Model file for the job. Use its own axes, mm. A direction names the side the tool comes from. Give positions to 0.01 mm unless a question says otherwise; leave off trailing zeros. Write each loop counter-clockwise with the first axis right and the second up, starting at its lowest first coordinate (ties: lowest second). Pieces come first, ordered by that corner, then holes. Notation, with made-up numbers: (-17.75, 36) - (-13.75, 36) arc R22 ccw to (-13.75, 42) - close; hole circle Ø3 at (4, -1). An arc over 180 degrees is marked (long way). Use a Markdown table: item, result. Add a question column.
Autodesk Inventor part; units mm, degrees
ref_plane "YZ Plane" through (0, 0, 0) normal (1, 0, 0) x (0, 1, 0)
ref_plane "XZ Plane" through (0, 0, 0) normal (0, 1, 0) x (-1, 0, 0)
ref_plane "XY Plane" through (0, 0, 0) normal (0, 0, 1) x (1, 0, 0)
sketch "Sketch1" plane through (0, 0, 0) normal (0, 0, 1) x (1, 0, 0)
  line L0 (-18.415, 5.9563) -> (18.415, 5.9563)
  line L1 (18.415, 5.9563) -> (18.415, -5.9563)
  line L2 (18.415, -5.9563) -> (-18.415, -5.9563)
  line L3 (-18.415, -5.9563) -> (-18.415, 5.9563)
  line L4 (-18.415, 5.9563) -> (18.415, -5.9563) construction
  line L5 (18.415, 5.9563) -> (-18.415, -5.9563) construction
  point P0 (0, 0)
  dimension "d0" = 36.83
  dimension "d1" = 11.9126
extrude "Extrusion1" add sketch "Sketch1" along normal blind 6.35
sketch "Sketch2" plane through (0, 0, 6.35) normal (0, 0, 1) x (1, 0, 0)
  line L0 (-18.415, 5.9563) -> (-18.415, -5.9563)
  line L1 (-18.415, 0) -> (18.415, 0)
  line L2 (18.415, -5.9563) -> (18.415, 5.9563)
  line L3 (-18.415, 0) -> (-20.6375, 0)
  line L4 (-18.415, 0) -> (-12.065, 0)
  circle A0 centre (-12.065, 0) radius 2.3241
  circle A1 centre (0.635, 0) radius 2.3241
  circle A2 centre (13.335, 0) radius 2.3241
  line L5 (-13.716, 2.286) -> (-10.414, 2.286)
  line L6 (-9.779, 1.651) -> (-9.779, -1.651)
  line L7 (-10.414, -2.286) -> (-13.716, -2.286)
  line L8 (-14.351, -1.651) -> (-14.351, 1.651)
  line L9 (-14.351, 2.286) -> (-9.779, -2.286) construction
  line L10 (-9.779, 2.286) -> (-14.351, -2.286) construction
  line L11 (11.684, 2.286) -> (14.986, 2.286)
  line L12 (15.621, 1.651) -> (15.621, -1.651)
  line L13 (14.986, -2.286) -> (11.684, -2.286)
  line L14 (11.049, -1.651) -> (11.049, 1.651)
  line L15 (11.049, 2.286) -> (15.621, -2.286) construction
  line L16 (15.621, 2.286) -> (11.049, -2.286) construction
  arc A3 (-13.716, 2.286) -> (-14.351, 1.651) centre (-13.716, 1.651) ccw
  arc A4 (-9.779, 1.651) -> (-10.414, 2.286) centre (-10.414, 1.651) ccw
  arc A5 (-10.414, -2.286) -> (-9.779, -1.651) centre (-10.414, -1.651) ccw
  arc A6 (-14.351, -1.651) -> (-13.716, -2.286) centre (-13.716, -1.651) ccw
  arc A7 (11.684, 2.286) -> (11.049, 1.651) centre (11.684, 1.651) ccw
  arc A8 (15.621, 1.651) -> (14.986, 2.286) centre (14.986, 1.651) ccw
  arc A9 (14.986, -2.286) -> (15.621, -1.651) centre (14.986, -1.651) ccw
  arc A10 (11.049, -1.651) -> (11.684, -2.286) centre (11.684, -1.651) ccw
  point P0 (0, 0)
  point P1 (-9.779, -0.4191)
  point P2 (-9.7409, 0)
  point P3 (-9.779, 0)
  dimension "d5" = 6.35
  dimension "d6" = 4.6482
  dimension "d9" = 12.7
  dimension "d16" = 4.572
  dimension "d17" = 4.572
  dimension "d18" = 4.572
  dimension "d19" = 4.572
  dimension "d20" = 0.635
extrude "Extrusion2" add sketch "Sketch2" along normal blind 1.5875 contours L8 A0 L5 L6 L1 | L1 L6 A0 L7 L8 | L8 A3 L5 A0 | A0 L7 A6 L8 | L1 A0 L6 | L5 A4 L6 A0 | A0 L6 A5 L7 | L14 A2 L11 L12 L1 | L1 L12 A2 L13 L14 | L14 A7 L11 A2 | A2 L13 A10 L14 | A2 L11 A8 L12 | L12 A9 L13 A2 picked at (-9.772, -0.2331)
extrude "Extrusion3" cut sketch "Sketch2" against normal through all contours A1 L1 | L1 A1
sketch "Sketch9" plane through (-18.415, 5.9563, 0) normal (0, 1, 0) x (1, 0, 0)
  line L0 (0, 0) -> (36.83, 0)
  line L1 (0, -6.35) -> (36.83, -6.35)
  line L2 (0, 0) -> (22.225, 0)
  line L3 (22.225, 0) -> (22.225, -6.35)
  line L4 (22.225, -6.35) -> (0, -6.35)
  line L5 (0, -6.35) -> (0, 0)
  point P0 (18.415, 0)
  dimension "d45" = 22.225
extrude "Extrusion9" add sketch "Sketch9" along normal blind 24.13
sketch "Sketch10" plane through (0, 0, 0) normal (0, 0, -1) x (-1, 0, 0)
  line L0 (-18.415, 5.9563) -> (-3.81, 5.9563)
  line L1 (18.415, 30.0863) -> (-3.81, 30.0863)
  arc A0 (-3.81, 5.9563) -> (-3.81, 30.0863) centre (-3.81, 18.0213) ccw
  line L2 (-3.81, 30.0863) -> (-3.81, 5.9563)
  point P0 (0, 0)
extrude "Extrusion10" cut sketch "Sketch10" against normal blind 19.05
fillet "Fillet7" radius 0.381 1 edges at (3.81, 30.0863, 3.175)
fillet "Fillet8" radius 3.175 4 edges at (-18.415, 30.0863, 3.175) (18.415, 5.9563, 3.175) (18.415, -5.9563, 3.175) (-18.415, -5.9563, 3.175)
sketch "Sketch11" plane through (0, 0, 0) normal (0, 0, -1) x (-1, 0, 0)
  circle A0 centre (-0.635, 0) radius 2.3241
  circle A1 centre (-0.635, 0) radius 4.1275
  point P0 (0, 0)
  dimension "d52" = 8.255
extrude "Extrusion11" cut sketch "Sketch11" against normal blind 3.175
properties part number "piston holder for goal rush"
(1) Band-saw the part on C-C (x = 13.5). Write the cut outline in (y, z), then the cut area to 3 significant figures.
(2) Band-saw the part on A-A (x = -1). Write the cut outline in (y, z) (3 decimals), then the cut area to 3 significant figures.
(3) Flat gauge pins, fed straight in: pin 1 (0.8 mm diameter, centred on y = -0.5, z = 7.5, fed in from +X); pin 2 (6.5 mm diameter, centred on x = 0.635, y = 0, fed in from -Z) (3 decimals); pin 3 (1.3 mm diameter, centred on x = 13, z = 7.5, fed in from +Y). Where does each tip first touch, or does it go through?
(4) Which spindle directions (+Z, -Z, +X, -X, +Y, -Y) get a long thin tool onto all of the face, cutting with end or side? Do faces 5 (the flat face through (-12, 2.286, 7)), 6 (the flat face through (-9.779, -1, 7)), 7 (the flat face through (11.049, 0, 7)). Say none if no direction does.
(5) Probe probe 1 along X at (y, z) = (0, 5.3) (3 decimals); probe 2 along X at (y, z) = (1.5, 7.25); probe 3 along Y at (x, z) = (9, 6.25). List the from-to ranges inside material, lowest first. Write a range as [from, to].
(6) Two-plate mould, pull along Y, no slides. Class faces 1 (the flat face through (-12, -2.286, 7)), 2 (the cylindrical face through (17.51, 5, 3.22)), 3 (the cylindrical face through (0.13, -2.27, 4.78)), 4 (the flat face through (13, 0, 7.938)): +Y half, -Y half, draft (parallel to the pull), parting line (faces both ways), or undercut.
Model answer:
| question | item | result |
|---|---|---|
| 1 | outline | (-5.96, 0) - (5.96, 0) - (5.96, 6.35) - (2.29, 6.35) - (2.29, 7.94) - (-2.29, 7.94) - (-2.29, 6.35) - (-5.96, 6.35) - close |
| 1 | area | 82.9 mm^2 |
| 2 | outline | (-5.956, 0) - (-3.79, 0) - (-3.79, 3.175) - (-1.652, 3.175) - (-1.652, 6.35) - (-5.956, 6.35) - close; (1.652, 3.175) - (3.79, 3.175) - (3.79, 0) - (6.957, 0) - (6.957, 6.35) - (1.652, 6.35) - close; (29.086, 0) - (30.086, 0) - (30.086, 6.35) - (29.086, 6.35) - close |
| 2 | area | 53.8 mm^2 |
| 3 | pin 1 | stops at x = 15.62 |
| 3 | pin 2 | stops at z = 3.175 |
| 3 | pin 3 | stops at y = 2.29 |
| 4 | face 5 | +Z, +X, -X, +Y |
| 4 | face 6 | +Z, -Y |
| 4 | face 7 | +Z, +Y, -Y |
| 5 | probe 1 | x = [-18.415, -1.689], [2.959, 18.415] |
| 5 | probe 2 | x = [-14.35, -9.78], [11.05, 15.62] |
| 5 | probe 3 | y = [-5.96, 5.96] |
| 6 | face 1 | -Y half |
| 6 | face 2 | +Y half |
| 6 | face 3 | undercut |
| 6 | face 4 | draft |
